```python
from build123d import *

# Parameters (mm, degrees)
SALIENTE_EXTRUIR1_DEPTH = 10
CROQUIS2_R              = 1.9
CORTAR_EXTRUIR1_DEPTH   = 25
CROQUIS5_R              = 3.25
CORTAR_EXTRUIR3_DEPTH   = 4
CORTAR_EXTRUIR4_DEPTH   = 4.25


with BuildPart() as part:
    # Croquis1 → Saliente-Extruir1 (new body)
    with BuildSketch(Plane.XY):
        with BuildLine():
            Line((65.8, 9.3), (-65.8, 9.3))
            ThreePointArc((-65.8, 9.3), (-70.042640687, 7.542640687), (-71.8, 3.3))
            Line((-71.8, 3.3), (-71.8, -3.3))
            ThreePointArc((-71.8, -3.3), (-70.042640687, -7.542640687), (-65.8, -9.3))
            Line((-65.8, -9.3), (-48.2, -9.3))
            Line((-48.2, -9.3), (-48.2, -1.5))
            Line((-48.2, -1.5), (-58.470111664, -1.5))
            ThreePointArc((-58.470111664, -1.5), (-66.8, 0), (-58.470111664, 1.5))
            Line((-58.470111664, 1.5), (-46.2, 1.5))
            Line((-46.2, 1.5), (-46.2, -9.3))
            Line((-46.2, -9.3), (46.2, -9.3))
            Line((46.2, -9.3), (46.2, 1.5))
            Line((46.2, 1.5), (58.470111664, 1.5))
            ThreePointArc((58.470111664, 1.5), (63.262063041, 4.231933355), (66.8, 0))
            ThreePointArc((66.8, 0), (63.262063041, -4.231933355), (58.470111664, -1.5))
            Line((58.470111664, -1.5), (48.2, -1.5))
            Line((48.2, -1.5), (48.2, -9.3))
            Line((48.2, -9.3), (65.8, -9.3))
            ThreePointArc((65.8, -9.3), (70.042640687, -7.542640687), (71.8, -3.3))
            Line((71.8, -3.3), (71.8, 3.3))
            ThreePointArc((71.8, 3.3), (70.042640687, 7.542640687), (65.8, 9.3))
        make_face()
    extrude(amount=SALIENTE_EXTRUIR1_DEPTH)

    # Croquis2 → Cortar-Extruir1 (cut, symmetric)
    with BuildSketch(Plane.XZ.offset(-1.5)):
        with Locations(Location((-53.335111664, 5, 0), (0, 0, 180))):
            Circle(CROQUIS2_R)
        with Locations(Location((53.335111664, 5, 0), (0, 0, 180))):
            Circle(CROQUIS2_R)
    extrude(amount=CORTAR_EXTRUIR1_DEPTH, both=True, mode=Mode.SUBTRACT)

    # Croquis5 → Cortar-Extruir3 (cut)
    with BuildSketch(Plane(origin=(0, 9.3, 0), x_dir=(1, 0, 0), z_dir=(0, 1, 0))):
        with Locations(Location((-53.335111664, -5, 0), (0, 0, 270))):
            Circle(CROQUIS5_R)
        with Locations(Location((53.335111664, -5, 0), (0, 0, 270))):
            Circle(CROQUIS5_R)
    extrude(amount=-CORTAR_EXTRUIR3_DEPTH, mode=Mode.SUBTRACT)

    # Croquis6 → Cortar-Extruir4 (cut)
    with BuildSketch(Plane(origin=(0, -9.3, 0), x_dir=(-1, 0, 0), z_dir=(0, -1, 0))):
        Polygon((49.871010049, -5), (51.603060857, -8), (55.067162472, -8), (56.799213279, -5), (55.067162472, -2), (51.603060857, -2), align=None)
        Polygon((-49.871010049, -5), (-51.603060857, -2), (-55.067162472, -2), (-56.799213279, -5), (-55.067162472, -8), (-51.603060857, -8), align=None)
    extrude(amount=-CORTAR_EXTRUIR4_DEPTH, mode=Mode.SUBTRACT)


solid = part.part
```
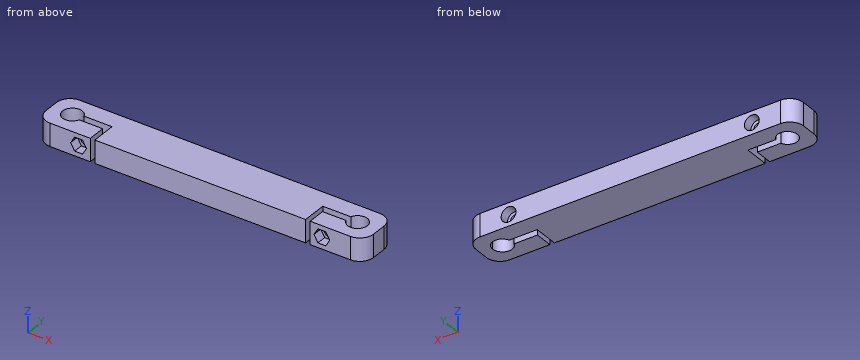
Can you work these out from the model? Positions are in its coordinate system, mm. Coordinates: 2 decimals unless noted, no trailing zeros. Order: outer loops, then holes, each group sorted by start corner. A loop starts at its lowest first (then second) coordinate and runs counter-clockwise, first axis right, second up.
1. I'm going to push flat-ended pins straight in: pin 1 (6 mm diameter, centred on x = -53.34, z = 5, fed in from +Y); pin 2 (6 mm diameter, centred on y = -7, z = 7.5, fed in from +X). Where does each tip first touch, or does it pass through?
2. If we section it at B-B (y = 6.75): Please give me the cut outline in (x, z), then the cut area to 3 significant figures.
3. If we section it at A-A (x = -62.5): Please give me the cut outline in (y, z).
4. I need wall thicknesses on line 1 (X direction, y = 0, z = 6.5); line 2 (Z direction, x = -53, y = -3.5); line 3 (X direction, y = 2.55, z = 5). Which ranges of each line are inside material? Lowest first, please.
Entries:
1. pin 1: stops at y = 5.3
1. pin 2: stops at x = 71.76
2. outline: (-70.71, 0) - (70.71, 0) - (70.71, 10) - (-70.71, 10) - close; hole circle Ø6.5 at (-53.34, 5); hole circle Ø6.5 at (53.34, 5)
2. area: 1,350 mm2
3. outline: (-9.3, 0) - (-4.3, 0) - (-4.3, 10) - (-9.3, 10) - close; (4.3, 0) - (9.3, 0) - (9.3, 10) - (4.3, 10) - close
4. line 1: x = -71.8 to -66.8, -46.2 to 46.2, 66.8 to 71.8
4. line 2: z = 0 to 3.13, 6.87 to 10
4. line 3: x = -71.8 to -65.96, -59.04 to -55.24, -51.44 to 51.44, 55.24 to 59.04, 65.96 to 71.8
